from build123d import *

# Parameters (mm, degrees)
EXTRUDE_1_DEPTH     = 5
SKETCH_4_R          = 1.6
CUT_EXTRUDE_1_DEPTH = 10
SKETCH_5_W          = 23
SKETCH_5_H          = 49
EXTRUDE_2_DEPTH     = 25
SHELL_1_T           = -2
SKETCH_6_R          = 6
SKETCH_6_W          = 14
SKETCH_6_H          = 7
CUT_EXTRUDE_2_DEPTH = 2
SKETCH_7_R          = 0.9
CUT_EXTRUDE_3_DEPTH = 5
SKETCH_10_R         = 0.9
CUT_EXTRUDE_4_DEPTH = 10
SKETCH_11_W         = 45
SKETCH_11_H         = 49
EXTRUDE_3_DEPTH     = 7


with BuildPart() as part:
    # Sketch 2 → Extrude 1 (new body)
    with BuildSketch(Plane(origin=(0, 0, 0), x_dir=(1, 0, 0), z_dir=(0, 1, 0))):
        with BuildLine():
            Line((6, -39.466401061), (6, -33.466401061))
            ThreePointArc((6, -33.466401061), (26.076809621, -21.817424229), (34, 0))
            Line((34, 0), (34, 51))
            Line((34, 51), (11, 51))
            Line((11, 51), (11, 100))
            Line((11, 100), (-34, 100))
            Line((-34, 100), (-34, 0))
            ThreePointArc((-34, 0), (-26.076809621, -21.817424229), (-6, -33.466401061))
            Line((-6, -33.466401061), (-6, -39.466401061))
            Line((-6, -39.466401061), (-2, -39.466401061))
            Line((-2, -39.466401061), (-2, -29.933259094))
            ThreePointArc((-2, -29.933259094), (0, 30), (2, -29.933259094))
            Line((2, -29.933259094), (2, -39.466401061))
            Line((2, -39.466401061), (6, -39.466401061))
        make_face()
        with BuildLine():
            ThreePointArc((-0.65, 90), (1, 88.35), (2.65, 90))
            Line((2.65, 90), (2.65, 95))
            ThreePointArc((2.65, 95), (1, 96.65), (-0.65, 95))
            Line((-0.65, 95), (-0.65, 90))
        make_face(mode=Mode.SUBTRACT)
        with BuildLine():
            ThreePointArc((-31.65, 90), (-30, 88.35), (-28.35, 90))
            Line((-28.35, 90), (-28.35, 95))
            ThreePointArc((-28.35, 95), (-30, 96.65), (-31.65, 95))
            Line((-31.65, 95), (-31.65, 90))
        make_face(mode=Mode.SUBTRACT)
        with BuildLine():
            ThreePointArc((-27.5, 74.5), (-14.5, 61.5), (-1.5, 74.5))
            Line((-1.5, 74.5), (-1.5, 79.5))
            ThreePointArc((-1.5, 79.5), (-14.5, 92.5), (-27.5, 79.5))
            Line((-27.5, 79.5), (-27.5, 74.5))
        make_face(mode=Mode.SUBTRACT)
        with BuildLine():
            ThreePointArc((-0.65, 59), (1, 57.35), (2.65, 59))
            Line((2.65, 59), (2.65, 64))
            ThreePointArc((2.65, 64), (1, 65.65), (-0.65, 64))
            Line((-0.65, 64), (-0.65, 59))
        make_face(mode=Mode.SUBTRACT)
        with BuildLine():
            ThreePointArc((-31.65, 59), (-30, 57.35), (-28.35, 59))
            Line((-28.35, 59), (-28.35, 64))
            ThreePointArc((-28.35, 64), (-30, 65.65), (-31.65, 64))
            Line((-31.65, 64), (-31.65, 59))
        make_face(mode=Mode.SUBTRACT)
    extrude(amount=EXTRUDE_1_DEPTH)

    # Sketch 4 → Cut-Extrude 1 (cut, symmetric)
    with BuildSketch(Plane(origin=(0, 0, 0), x_dir=(0, 0, -1), z_dir=(1, 0, 0))):
        with Locations((-36.466401061, 2.5)):
            Circle(SKETCH_4_R)
    extrude(amount=CUT_EXTRUDE_1_DEPTH, both=True, mode=Mode.SUBTRACT)



with BuildPart() as body_2:
    # Sketch 5 → Extrude 2 (new body)
    with BuildSketch(Plane(origin=(0, 0, 0), x_dir=(1, 0, 0), z_dir=(0, 1, 0))):
        with Locations((22.5, 75.5)):
            Rectangle(SKETCH_5_W, SKETCH_5_H)
    extrude(amount=EXTRUDE_2_DEPTH)

    # Shell 1
    shell_1_openings = [body_2.faces().sort_by_distance(p)[0] for p in [
        (22.5, 25, -75.5),
    ]]
    offset(amount=SHELL_1_T, openings=shell_1_openings, kind=Kind.INTERSECTION)

    # Sketch 6 → Cut-Extrude 2 (cut)
    with BuildSketch(Plane(origin=(0, 0, -100), x_dir=(-1, 0, 0), z_dir=(0, 0, -1))):
        with Locations((-22.5, 17)):
            Circle(SKETCH_6_R)
        with Locations((-22.5, 6)):
            Rectangle(SKETCH_6_W, SKETCH_6_H)
    extrude(amount=-CUT_EXTRUDE_2_DEPTH, mode=Mode.SUBTRACT)

    # Sketch 7 → Cut-Extrude 3 (cut)
    with BuildSketch(Plane(origin=(0, 25, 0), x_dir=(1, 0, 0), z_dir=(0, 1, 0))):
        with Locations((12.717157288, 52.717157288)):
            Circle(SKETCH_7_R)
        with Locations((32.282842712, 52.717157288)):
            Circle(SKETCH_7_R)
        with Locations((32.282842712, 98.282842712)):
            Circle(SKETCH_7_R)
        with Locations((12.717157288, 98.282842712)):
            Circle(SKETCH_7_R)
    extrude(amount=-CUT_EXTRUDE_3_DEPTH, mode=Mode.SUBTRACT)

    # Sketch 10 → Cut-Extrude 4 (cut)
    with BuildSketch(Plane(origin=(0, 2, 0), x_dir=(1, 0, 0), z_dir=(0, 1, 0))):
        with Locations(Location((15, 95.75, 0), (0, 0, 270))):
            Circle(SKETCH_10_R)
        with Locations(Location((30, 95.75, 0), (0, 0, 90))):
            Circle(SKETCH_10_R)
        with Locations(Location((30, 55.25, 0), (0, 0, 270))):
            Circle(SKETCH_10_R)
        with Locations(Location((15, 55.25, 0), (0, 0, 90))):
            Circle(SKETCH_10_R)
    extrude(amount=-CUT_EXTRUDE_4_DEPTH, mode=Mode.SUBTRACT)


with BuildPart() as part_1:
    add(part.part)

    add(body_2.part)  # Extrude 3 merges body 2
    # Sketch 11 → Extrude 3 (add)
    with BuildSketch(Plane(origin=(0, 5, 0), x_dir=(1, 0, 0), z_dir=(0, 1, 0))):
        with Locations((-11.5, 75.5)):
            Rectangle(SKETCH_11_W, SKETCH_11_H)
        with BuildLine():
            Line((-0.65, 95), (-0.65, 90))
            ThreePointArc((-0.65, 90), (1, 88.35), (2.65, 90))
            Line((2.65, 90), (2.65, 95))
            ThreePointArc((2.65, 95), (1, 96.65), (-0.65, 95))
        make_face(mode=Mode.SUBTRACT)
        with BuildLine():
            Line((-31.65, 95), (-31.65, 90))
            ThreePointArc((-31.65, 90), (-30, 88.35), (-28.35, 90))
            Line((-28.35, 90), (-28.35, 95))
            ThreePointArc((-28.35, 95), (-30, 96.65), (-31.65, 95))
        make_face(mode=Mode.SUBTRACT)
        with BuildLine():
            Line((-27.5, 79.5), (-27.5, 74.5))
            ThreePointArc((-27.5, 74.5), (-14.5, 61.5), (-1.5, 74.5))
            Line((-1.5, 74.5), (-1.5, 79.5))
            ThreePointArc((-1.5, 79.5), (-14.5, 92.5), (-27.5, 79.5))
        make_face(mode=Mode.SUBTRACT)
        with BuildLine():
            Line((-0.65, 64), (-0.65, 59))
            ThreePointArc((-0.65, 59), (1, 57.35), (2.65, 59))
            Line((2.65, 59), (2.65, 64))
            ThreePointArc((2.65, 64), (1, 65.65), (-0.65, 64))
        make_face(mode=Mode.SUBTRACT)
        with BuildLine():
            Line((-31.65, 64), (-31.65, 59))
            ThreePointArc((-31.65, 59), (-30, 57.35), (-28.35, 59))
            Line((-28.35, 59), (-28.35, 64))
            ThreePointArc((-28.35, 64), (-30, 65.65), (-31.65, 64))
        make_face(mode=Mode.SUBTRACT)
    extrude(amount=EXTRUDE_3_DEPTH)


solid = part_1.part
Source: CAD feature listing. Evaluate the final solid. Frame: model axes, mm. A direction names the side the tool comes from. Coordinates: 2 decimals unless noted, no trailing zeros. Write each loop counter-clockwise with the first axis right and the second up, starting at its lowest first coordinate (ties: lowest second). Pieces come first, ordered by that corner, then holes. Notation, with made-up numbers: M 45.5,48 L 72.5,48 A18 cw 72.5,65 Z; hole C 65.5,-20 d11. An arc over 180 degrees is marked long. Use a Markdown table: item, result.
1) Ray query, L1, parallel to X at y = 6.75, z = -80; L2, parallel to X at y = 0.45, z = -55.25; L3, parallel to X at y = 16, z = -82.5. Return the intervals inside material, ascending.
Conclusion:
| item | result |
|---|---|
| L1 | x = -34 to -27.49, -1.51 to 13, 32 to 34 |
| L2 | x = -34 to 14.1, 15.9 to 29.1, 30.9 to 34 |
| L3 | x = 11 to 13, 32 to 34 |
2) Section A-A, the plane y = 7.5. Give the number of separate pieces and of enclosed holes in the cut face, then the cut area to 3 significant figures.
Conclusion:
| item | result |
|---|---|
| separate pieces | 1 |
| enclosed holes | 5 |
| area | 1,690 mm^2 |
3) First-contact query: pin 1 Ø2 at (x, z) = (15, -95.75) entering from +Y; pin 2 Ø1 at (x, z) = (0.5, -37.5) entering from +Y; pin 3 Ø1.5 at (x, y) = (-4, 11.5) entering from +Z; pin 4 Ø2.5 at (y, z) = (2.5, 36.5) entering from -X. Flat tips, straight axial feed; report the tip coordinate or a pass-through.
Conclusion:
| item | result |
|---|---|
| pin 1 | stops at y = 2 |
| pin 2 | stops at y = 5 |
| pin 3 | stops at z = -51 |
| pin 4 | passes through |
4) Section C-C, the plane z = -12.5. Output: boundary loops of the cut face in (x, y).
Conclusion:
| item | result |
|---|---|
| outline | M -34,0 L -27.27,0 L -27.27,5 L -34,5 Z; M 27.27,0 L 34,0 L 34,5 L 27.27,5 Z |
5) Mould query, pull axis Z, two halves, no side actions, for faces 4 (the flat face through (11, 18, -75)), 5 (the flat face through (7, 10, -51)), 6 (the cylindrical face through (-29.96, 5.92, -96.65)). Classes: pulls with the +Z half, pulls with the -Z half, needs draft (parallel to the pull), parting line crosses it, or undercut.
Conclusion:
| item | result |
|---|---|
| face 4 | needs draft |
| face 5 | pulls with the +Z half |
| face 6 | undercut |
6) Reachability of faces 1 (the flat face through (22, 13, -53)), 2 (the flat face through (6, 1, 38)), 3 (the cylindrical face through (1.04, 5.92, -96.65)) from +Z, -Z, +X, -X, +Y, -Y: full face, straight path, thin tool, end or side. Return the list, or none.
Conclusion:
| item | result |
|---|---|
| face 1 | +Y |
| face 2 | +Z, +X, +Y, -Y |
| face 3 | +Y, -Y |
7) Section B-B, the plane x = 25. Output: boundary loops of the cut face in (y, z).
Conclusion:
| item | result |
|---|---|
| outline | M 0,-100 L 2.5,-100 L 2.5,-98 L 2,-98 L 2,-53 L 25,-53 L 25,-51 L 5,-51 L 5,-16.58 L 0,-16.58 Z; M 0,16.58 L 5,16.58 L 5,23.04 L 0,23.04 Z; M 9.5,-100 L 11.55,-100 L 11.55,-98 L 9.5,-98 Z; M 22.45,-100 L 25,-100 L 25,-98 L 22.45,-98 Z |
8) Section D-D, the plane x = -4. Output: boundary loops of the cut face in (y, z).
Conclusion:
| item | result |
|---|---|
| outline | M 0,-100 L 12,-100 L 12,-87.16 L 0,-87.16 Z; M 0,-66.84 L 12,-66.84 L 12,-51 L 5,-51 L 5,-29.73 L 0,-29.73 Z; M 0,29.73 L 5,29.73 L 5,39.47 L 0,39.47 Z; hole C 2.5,36.47 d3.2 |
